```python
from build123d import *

# Parameters (mm, degrees)
CHAMFER1_SIZE      = 1
SKETCH2_OUTSIDE_W  = 28.378
SKETCH2_OUTSIDE_H  = 28.378
CUT_EXTRUDE1_DEPTH = 3.3
CHAMFER2_SIZE      = 0.2


with BuildPart() as part:
    # Sketch1 → Revolve1 (revolve)
    with BuildSketch(Plane.XY, mode=Mode.PRIVATE) as revolve1_sk:
        Polygon((0, 0), (5.975, 0), (5.975, 13.6), (4.785, 13.6), (4.785, 16.5), (6.265, 16.5), (6.265, 20.3), (8.22, 20.3), (8.22, 25.4), (3.5, 25.4), (3.5, 37), (5.5, 39), (5.5, 41), (3.814137214, 43.92), (0, 43.92), align=None)
    revolve(revolve1_sk.sketch.rotate(Axis((0, 0, 0), (0, 1, 0)), 90), axis=Axis((0, 0, 0), (0, 1, 0)))

    # Chamfer1
    chamfer1_edges = [part.edges().sort_by_distance(p)[0] for p in [
        (0, 13.6, 5.975),
        (0, 0, 5.975),
    ]]
    chamfer(chamfer1_edges, length=CHAMFER1_SIZE)

    # Sketch2 outside → Cut-Extrude1 (cut)
    with BuildSketch(Plane(origin=(0, 25.4, 0), x_dir=(1, 0, 0), z_dir=(0, 1, 0))):
        Rectangle(SKETCH2_OUTSIDE_W, SKETCH2_OUTSIDE_H)
        with BuildLine():
            Line((6.515, -5.012302365), (6.515, 5.012302365))
            ThreePointArc((6.515, 5.012302365), (0, 8.22), (-6.515, 5.012302365))
            Line((-6.515, 5.012302365), (-6.515, -5.012302365))
            ThreePointArc((-6.515, -5.012302365), (0, -8.22), (6.515, -5.012302365))
        make_face(mode=Mode.SUBTRACT)
    extrude(amount=-CUT_EXTRUDE1_DEPTH, mode=Mode.SUBTRACT)

    # Chamfer2
    chamfer2_edges = [part.edges().sort_by_distance(p)[0] for p in [
        (0, 25.4, 3.5),
        (0, 20.3, 8.22),
        (0, 20.3, 6.265),
        (0, 25.4, 8.22),
        (-3.630927881, 25.4, -7.374602547),
        (6.515, 25.4, 0),
        (-6.515, 25.4, 0),
    ]]
    chamfer(chamfer2_edges, length=CHAMFER2_SIZE)


solid = part.part
```
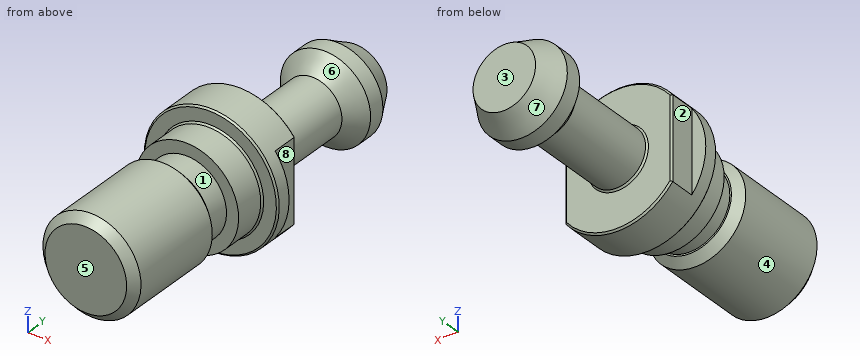
Geometry: final body of the model. Coordinates: model frame, mm. Face numbers are marked on the shaded views. A direction names the side the tool comes from. Round coordinates to 2 decimals unless told otherwise and drop trailing zeros. Write each loop counter-clockwise with the first axis right and the second up, starting at its lowest first coordinate (ties: lowest second). Pieces come first, ordered by that corner, then holes. Notation, with made-up numbers: (64, -30) -> (68, -30) arc R31 cw to (68, -4) -> close; hole circle Ø4 at (21, 89.5). An arc over 180 degrees is marked (long way). Use CSV: the item, a comma, the result in double quotes. Start each with the question number.
Q1. First-contact query: pin 1 Ø5 at (x, y) = (-5.5, 36.5) entering from -Z; pin 2 Ø1.9 at (x, z) = (7.5, -2) entering from +Y; pin 3 Ø1 at (y, z) = (11, -5.5) entering from -X. Flat tips, straight axial feed; report the tip coordinate or a pass-through.
Q2. Reachability of the marked faces 1, 2, 3 and 4 from +Z, -Z, +X, -X, +Y, -Y: full face, straight path, thin tool, end or side. Return the list, or none.
Q3. Section A-A (y = 38). Return loops of the section in (x, z).
Q4. Line query: L1, parallel to Y at x = -3.5, z = -3.5; L2, parallel to Y at x = -7.25, z = 2.5; L3, parallel to Y at x = 5.75, z = -2. Output: solid intervals per line, ascending.
Q5. Pull-direction query (Y, two-part tool) for the marked faces 5, 6, 7 and 8; classes: pulls with the +Y half, pulls with the -Y half, needs draft (parallel to the pull), parting line crosses it, or undercut.
Q6. Section B-B (y = 15). Return loops of the section in (x, z) (3 decimals).
Result sheet:
1,pin 1,"z = -3"
1,pin 2,"y = 22.1"
1,pin 3,"x = -3.27"
2,face 1,"none"
2,face 2,"+Z, -Z, -X, +Y"
2,face 3,"+Z, -Z, +X, -X, +Y"
2,face 4,"-Y"
3,outline,"circle Ø9 at (0, 0)"
4,L1,"0 to 13.6, 16.5 to 25.4, 38.45 to 41.95"
4,L2,"20.3 to 22.1"
4,L3,"16.5 to 25.4"
5,face 5,"pulls with the -Y half"
5,face 6,"undercut"
5,face 7,"pulls with the +Y half"
5,face 8,"needs draft"
6,outline,"circle Ø9.57 at (0, 0)"
